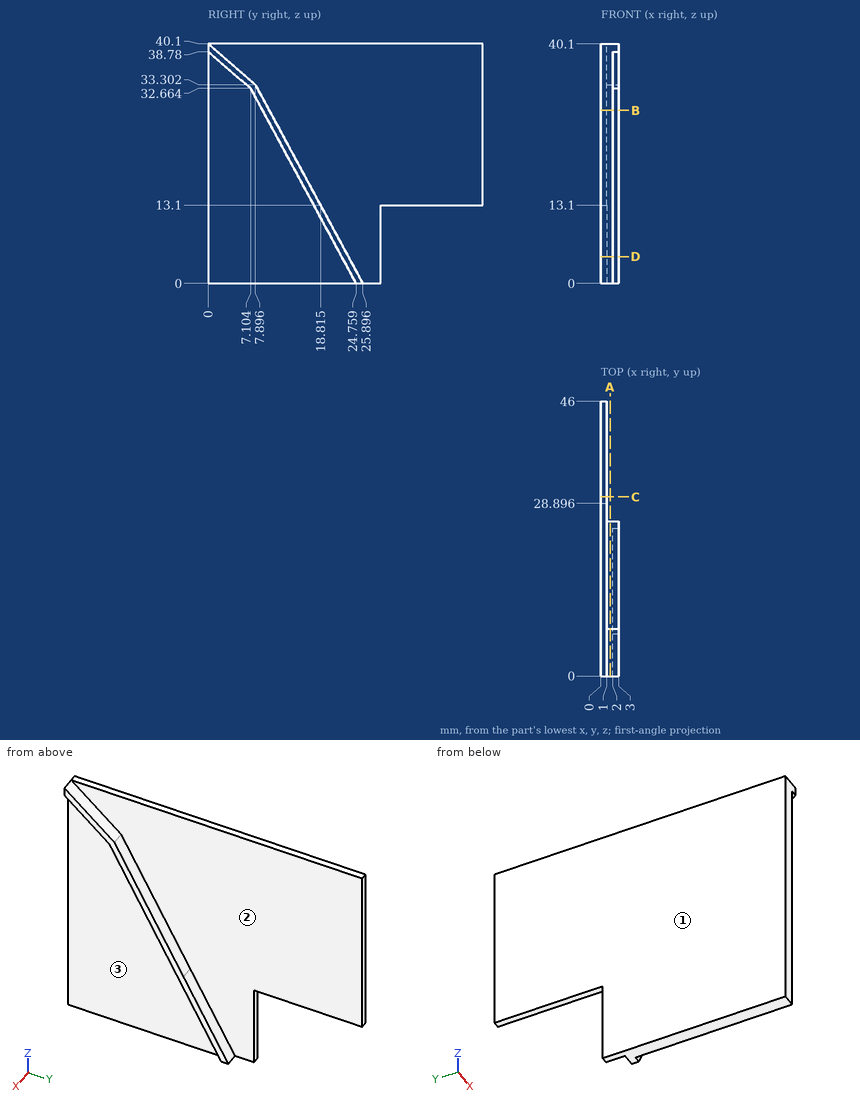
Part print with two shaded views. Sizes in mm from the minimum x, y, z corner. A direction names the side the tool comes from. Give positions to 0.01 mm unless a question says otherwise; leave off trailing zeros. Order: outer loops, then holes, each group sorted by start corner. A loop starts at its lowest first (then second) coordinate and runs counter-clockwise, first axis right, second up. Notation, with made-up numbers: (42, -21.75) - (53, -21.75) arc R31 cw to (53, 6.25) - close; hole circle Ø2 at (26, 49.5). An arc over 180 degrees is marked (long way). Write each question's results on one line, items separated by ' | '.
1. Saw through at B-B on z = 29. List the corners of the cut face in (x, y) (1 decimal).
Calculated:
outline: (0, 0) - (2, 0) - (2, 9.1) - (3, 9.1) - (3, 10.2) - (1, 10.2) - (1, 46) - (0, 46) - close
2. Probe L1, parallel to X at y = 35.5, z = 28.5; L2, parallel to Y at x = 0.75, z = 5; L3, parallel to X at y = 5.5, z = 29.5. List the from-to ranges inside material, lowest first. Write a range as from..to.
Calculated:
L1: x = 0..1 | L2: y = 0..28.9 | L3: x = 0..2
3. 3-axis set-ups, long thin cutter, end or side, ignore diameter. For the marked faces 1, 2 and 3: which of +Z, -Z, +X, -X, +Y, -Y reach the whole face in a straight line?
Calculated:
face 1: +Z, -Z, -X, +Y, -Y | face 2: +Z, +X, +Y | face 3: -Z, +X, -Y
4. Saw through at D-D on z = 4.5. List the corners of the cut face in (x, y).
Calculated:
outline: (0, 0) - (2, 0) - (2, 22.33) - (3, 22.33) - (3, 23.46) - (1, 23.46) - (1, 28.9) - (0, 28.9) - close
5. Pin check, flat tips, straight feed: pin 1 (0.8 mm diameter, centred on x = 0.5, z = 7.5, fed in from +Y); pin 2 (4 mm diameter, centred on y = 32.5, z = 8.5, fed in from +X); pin 3 (0.8 mm diameter, centred on x = 0.5, y = 40.5, fed in from -Z); pin 4 (4 mm diameter, centred on y = 14.5, z = 31, fed in from +X). Stop position of each tip, or through.
Calculated:
pin 1: stops at y = 28.9 | pin 2: passes through | pin 3: stops at z = 13.1 | pin 4: stops at x = 1
6. Saw through at C-C on y = 30. List the corners of the cut face in (x, z).
Calculated:
outline: (0, 13.1) - (1, 13.1) - (1, 40.1) - (0, 40.1) - close
7. Saw through at A-A on x = 1.55. List the corners of the cut face in (y, z) (1 decimal).
Calculated:
outline: (0, 0) - (25.9, 0) - (7.9, 33.3) - (0, 40.1) - close
